from build123d import *

# Parameters (mm, degrees)
MAIN_FACE_R                    = 1.5749999999999995
MAIN_FACE_R_2                  = 1.5750000000000013
MAIN_FACE_R_3                  = 11.5
MAINFACE_DEPTH                 = 7.5
SKETCH2_W                      = 7.500000000000001
SKETCH2_H                      = 42.30000000000015
SIDEPROFILE_DEPTH              = 11
NON_INTERFERING_FILLET_DEPTH   = 67.5049810164623
BASECLEARANCE_DEPTH            = 1.5
GROUDINGBOLTHOLES_DEPTH        = 68.46897435117894
GROUDINGBOLTHOLES_DEPTH_BACK   = 68.46897435117894
SKETCH5_R                      = 1.5749999999999995
BOLTACCESSHOLES_START          = -10
SKETCH5_3_R                    = 3.55
SKETCH5_3_R_2                  = 1.5749999999999995
SKETCH5_3_R_3                  = 3.5500000000000007
BOLTACCESSHOLES_DEPTH          = 47.50000000000001
HAPPYPRINTERCURVES_R           = 2
SKETCH6_W                      = 48.78690945060761
SKETCH6_H                      = 41.74981882727384
BASEPLATE_DEPTH                = 1.2
SUPPORTTORSIONBUTBREATHE_DEPTH = 67.6961957157231


with BuildPart() as part:
    # Main Face → MainFace (new body)
    with BuildSketch(Plane.XY):
        Polygon((0, 21.150000000000077), (21.150000000000077, 21.150000000000077), (21.150000000000087, 7.98e-14), (21.150000000000507, -21.149999999999572), (8.381e-14, -21.149999999999928), (-21.149999999999924, -21.149999999999928), (-21.149999999999995, -2.69e-15), (-21.149999999999856, 21.150000000000222), align=None)
        with Locations((15.499999999999996, 15.5)):
            Circle(MAIN_FACE_R, mode=Mode.SUBTRACT)
        with Locations((15.500000000000005, -15.500000000000002)):
            Circle(MAIN_FACE_R_2, mode=Mode.SUBTRACT)
        with Locations((-15.499999999999998, -15.500000000000012)):
            Circle(MAIN_FACE_R, mode=Mode.SUBTRACT)
        with Locations((-15.50000000000001, 15.49999999999999)):
            Circle(MAIN_FACE_R, mode=Mode.SUBTRACT)
        Circle(MAIN_FACE_R_3, mode=Mode.SUBTRACT)
    extrude(amount=MAINFACE_DEPTH)

    # Sketch2 → SideProfile (add)
    with BuildSketch(Plane.ZY.offset(21.149999999999995)):
        with Locations((3.7500000000000004, 2.1849e-13)):
            Rectangle(SKETCH2_W, SKETCH2_H)
        with BuildLine():
            Line((0, -21.14999999999986), (0, 21.150000000000293))
            Line((0, 21.150000000000293), (-1.771709500841494, 21.150000000000293))
            ThreePointArc((-1.7717095008414934, 21.150000000000297), (-5.828166751938932, 20.078151362319375), (-8.825687949345335, 17.14241097816094))
            ThreePointArc((-8.82568794934533, 17.142410978160935), (-20.697100679367818, 4.412586379453849), (-36.76838475660053, -2.2726737223876654))
            ThreePointArc((-36.76838475660055, -2.2726737223876654), (-39.086170348891756, -3.6262628829235943), (-40, -6.149999999999864))
            Line((-40, -6.149999999999864), (-40, -21.149999999999864))
            Line((-40, -21.149999999999864), (0, -21.149999999999856))
        make_face()
    sideprofile = extrude(amount=SIDEPROFILE_DEPTH)

    # Sketch3 → Non-interfering fillet (cut, symmetric)
    with BuildSketch(Plane(origin=(0, 21.150000000000077, 0), x_dir=(1, 0, 0), z_dir=(0, 1, 0))):
        with BuildLine():
            Line((-21.75000000000007, 0.5999999999999999), (-21.750000000000068, 41.938133152744264))
            Line((-21.750000000000068, 41.938133152744264), (-16.932175207311897, 41.938133152744264))
            Line((-16.932175207311897, 41.938133152744264), (-16.932175207311897, 2.9783080433489855))
            Line((-16.932175207311897, 2.9783080433489855), (-21.149999999999856, 0))
            ThreePointArc((-21.149999999999856, 0), (-21.574264068711923, 0.17573593128799603), (-21.75000000000007, 0.5999999999999999))
        make_face()
    non_interfering_fillet = extrude(amount=NON_INTERFERING_FILLET_DEPTH, both=True, mode=Mode.SUBTRACT)

    # Mirror1: SideProfile, Non-interfering fillet across plane
    add(sideprofile.mirror(Plane(origin=(0, 0, 0), x_dir=(0, 0, 1), z_dir=(1, 0, 0))))
    add(non_interfering_fillet.mirror(Plane(origin=(0, 0, 0), x_dir=(0, 0, 1), z_dir=(1, 0, 0))), mode=Mode.SUBTRACT)

    # Sketch4 → BaseClearance (add)
    with BuildSketch(Plane.XZ.offset(21.149999999999928)):
        with BuildLine():
            Line((21.749999999999716, -0.5999999999999999), (21.749999999999712, -39.99999999999999))
            Line((21.749999999999712, -39.99999999999999), (32.149999999999565, -40))
            Line((32.149999999999565, -40), (32.149999999999565, 7.5))
            Line((32.149999999999565, 7.5), (-32.150000000000276, 7.5))
            Line((-32.150000000000276, 7.5), (-32.150000000000276, -40))
            Line((-32.150000000000276, -40), (-21.750000000000433, -40))
            Line((-21.750000000000433, -40), (-21.75000000000043, -0.5999999999999998))
            ThreePointArc((-21.75000000000043, -0.5999999999999998), (-21.574264068712278, -0.17573593128799736), (-21.150000000000215, 0))
            Line((-21.150000000000215, 0), (21.149999999999498, 1.73e-15))
            ThreePointArc((21.149999999999498, 1.73e-15), (21.574264068711567, -0.17573593128799248), (21.749999999999716, -0.5999999999999999))
        make_face()
    extrude(amount=BASECLEARANCE_DEPTH)

    # Sketch5 → GroudingBoltHoles (cut, two sides: drawn at the far end of the back side and taken through both)
    with BuildSketch(Plane.XZ.offset(22.64999999999993).offset(-GROUDINGBOLTHOLES_DEPTH_BACK)):
        with Locations((-26.95000000000035, -4.0000000000000036)):
            Circle(SKETCH5_R)
        with Locations((-26.950000000000344, -34)):
            Circle(SKETCH5_R)
        with Locations((26.95000000000035, -33.99999999999999)):
            Circle(SKETCH5_R)
        with Locations((26.95000000000035, -3.9999999999999964)):
            Circle(SKETCH5_R)
    extrude(amount=GROUDINGBOLTHOLES_DEPTH + GROUDINGBOLTHOLES_DEPTH_BACK, mode=Mode.SUBTRACT)

    # Sketch5<3> → BoltAccessHoles (cut)
    # profile 1 of 4: a face of its own
    with BuildSketch(Plane.XZ.offset(22.64999999999993).offset(BOLTACCESSHOLES_START)):
        with Locations((-26.950000000000344, -34)):
            Circle(SKETCH5_3_R)
        with Locations((-26.950000000000344, -34)):
            Circle(SKETCH5_3_R_2, mode=Mode.SUBTRACT)
    # profile 2 of 4: a face of its own
    with BuildSketch(Plane.XZ.offset(22.64999999999993).offset(BOLTACCESSHOLES_START)):
        with Locations((-26.95000000000035, -4.0000000000000036)):
            Circle(SKETCH5_3_R_3)
    # profile 3 of 4: a face of its own
    with BuildSketch(Plane.XZ.offset(22.64999999999993).offset(BOLTACCESSHOLES_START)):
        with Locations(Location((26.95000000000035, -3.9999999999999964, 0), (0, 0, 38.879713196))):
            Circle(SKETCH5_3_R_3)
    # profile 4 of 4: a face of its own
    with BuildSketch(Plane.XZ.offset(22.64999999999993).offset(BOLTACCESSHOLES_START)):
        with Locations(Location((26.95000000000035, -33.99999999999999, 0), (0, 0, 308.755289776))):
            Circle(SKETCH5_3_R)
    extrude(amount=-BOLTACCESSHOLES_DEPTH, mode=Mode.SUBTRACT)

    # HappyPrinterCurves
    # the kernel refuses this fillet: 2 mm, written as the material it takes off along each edge
    with BuildSketch(Plane(origin=(32.1499999999999, -27.649999999999395, -40), x_dir=(0, 0, 1), z_dir=(1.29e-15, 1, 0))) as happyprintercurves_piece_1:
        with BuildLine():
            CenterArc((HAPPYPRINTERCURVES_R, -HAPPYPRINTERCURVES_R), HAPPYPRINTERCURVES_R, 90, 90)
            Line((0, -HAPPYPRINTERCURVES_R), (0, 0))
            Line((0, 0), (HAPPYPRINTERCURVES_R, 0))
        make_face()
    extrude(amount=26.49999999999942, mode=Mode.SUBTRACT)
    with BuildSketch(Plane(origin=(21.750000000000068, -1.1499999999999382, -40), x_dir=(0, 4.3e-16, 1), z_dir=(1.72e-15, -1, 4.3e-16))) as happyprintercurves_piece_2:
        with BuildLine():
            CenterArc((HAPPYPRINTERCURVES_R, -HAPPYPRINTERCURVES_R), HAPPYPRINTERCURVES_R, 90, 90)
            Line((0, -HAPPYPRINTERCURVES_R), (0, 0))
            Line((0, 0), (HAPPYPRINTERCURVES_R, 0))
        make_face()
    extrude(amount=26.49999999999963, mode=Mode.SUBTRACT)
    with BuildSketch(Plane(origin=(-32.149999999999984, -1.1499999999999737, -40), x_dir=(0, 0, 1), z_dir=(4.74e-15, -1, 0))) as happyprintercurves_piece_3:
        with BuildLine():
            CenterArc((HAPPYPRINTERCURVES_R, -HAPPYPRINTERCURVES_R), HAPPYPRINTERCURVES_R, 90, 90)
            Line((0, -HAPPYPRINTERCURVES_R), (0, 0))
            Line((0, 0), (HAPPYPRINTERCURVES_R, 0))
        make_face()
    extrude(amount=26.500000000000487, mode=Mode.SUBTRACT)
    with BuildSketch(Plane(origin=(-32.1499999999999, -27.65000000000046, 7.5), x_dir=(1, 3.89e-15, 0), z_dir=(-3.89e-15, 1, 0))) as happyprintercurves_piece_4:
        with BuildLine():
            CenterArc((HAPPYPRINTERCURVES_R, HAPPYPRINTERCURVES_R), HAPPYPRINTERCURVES_R, 180, 90)
            Line((0, HAPPYPRINTERCURVES_R), (0, 0))
            Line((0, 0), (HAPPYPRINTERCURVES_R, 0))
        make_face()
    extrude(amount=53.800000000000644, mode=Mode.SUBTRACT)
    with BuildSketch(Plane(origin=(-21.750000000000068, -27.65000000000029, -40), x_dir=(0, 0, 1), z_dir=(-1.08e-15, 1, 0))) as happyprintercurves_piece_5:
        with BuildLine():
            CenterArc((HAPPYPRINTERCURVES_R, -HAPPYPRINTERCURVES_R), HAPPYPRINTERCURVES_R, 90, 90)
            Line((0, -HAPPYPRINTERCURVES_R), (0, 0))
            Line((0, 0), (HAPPYPRINTERCURVES_R, 0))
        make_face()
    extrude(amount=26.500000000000348, mode=Mode.SUBTRACT)
    with BuildSketch(Plane(origin=(32.150000000000084, 26.150000000000183, 7.5), x_dir=(0, 0, -1), z_dir=(-2.6e-15, -1, 0))) as happyprintercurves_piece_6:
        with BuildLine():
            CenterArc((HAPPYPRINTERCURVES_R, -HAPPYPRINTERCURVES_R), HAPPYPRINTERCURVES_R, 90, 90)
            Line((0, -HAPPYPRINTERCURVES_R), (0, 0))
            Line((0, 0), (HAPPYPRINTERCURVES_R, 0))
        make_face()
    extrude(amount=53.79999999999958, mode=Mode.SUBTRACT)

    # Sketch6 → BasePlate (add)
    with BuildSketch(Plane.XZ.offset(22.64999999999993)):
        with Locations((-0.09860427356243306, -19.12509058636308)):
            Rectangle(SKETCH6_W, SKETCH6_H)
    extrude(amount=-BASEPLATE_DEPTH)

    # Sketch7 → SupportTorsionButBreathe (cut, through all)
    with BuildSketch(Plane(origin=(3.5542e-13, -21.449999999999932, 0), x_dir=(1, 1.657e-14, 0), z_dir=(-1.657e-14, 1, 0))):
        with BuildLine():
            Line((21.75000000000003, 36.768384756600554), (21.74999999999979, 26.401553875860724))
            ThreePointArc((21.74999999999979, 26.401553875860724), (-4e-15, 4.651553875860934), (-21.74999999999979, 26.401553875860724))
            Line((-21.74999999999979, 26.401553875860724), (-21.750000000000107, 36.76838475660055))
            Line((-21.750000000000107, 36.76838475660055), (-21.750000000000114, 38))
            ThreePointArc((-21.750000000000114, 38), (-22.335786437627018, 39.41421356237322), (-23.750000000000167, 40))
            Line((-23.750000000000167, 40), (-23.750000000000167, 46.1872525671472))
            Line((-23.750000000000167, 46.1872525671472), (23.749999999999964, 46.1872525671472))
            Line((23.749999999999964, 46.1872525671472), (23.749999999999964, 40))
            ThreePointArc((23.749999999999964, 40), (22.33578643762671, 39.414213562373185), (21.75000000000002, 38))
            Line((21.75000000000002, 38), (21.75000000000003, 36.768384756600554))
        make_face()
    extrude(amount=-SUPPORTTORSIONBUTBREATHE_DEPTH, mode=Mode.SUBTRACT)


solid = part.part
Read the model definition and answer for the solid it produces. Units are mm, in the model's axes. A direction names the side the tool comes from. Give positions to 0.01 mm unless a question says otherwise; leave off trailing zeros. Loops run counter-clockwise (first coordinate to the right, second up) from the corner with the lowest first, then second, coordinate; pieces in that order, holes last. Notation, with made-up numbers: (21.25, 71.5) - (48.25, 71.5) arc R7 ccw to (48.25, 77.5) - close; hole circle Ø7 at (8, 64.25). An arc over 180 degrees is marked (long way). Answer as CSV lines item,"result". Start each with the question number.
1) Which of the six approach directions +Z, -Z, +X, -X, +Y, -Y give full straight-line access (tool end or side, diameter ignored) to faces 1 (the face through (-25.042, 4.013, -1.007)), 2 (the face through (-25.448, -17.58, -3.527)), 3 (the face through (21.75, -5, -15))?
2) Straight lines are drawn through the part: L1, parallel to Z at x = -26.95, y = -15.25 (3 decimals); L2, parallel to X at y = -10.5, z = -11; L3, parallel to X at y = 13, z = -4. For each, find the intervals that lie inside material, in ascending order. Write a range as from..to.
3) Find section B-B (y = 8.5). Write down the section's boundary in (x, z), then the cut area to 3 significant figures.
4) Find section C-C (z = 4). Write down the section's boundary in (x, y) (3 decimals), then the cut area to 3 significant figures.
5) Each of these flat-tipped pins is pushed along its axis until it touches: pin 1 Ø12.5 at (x, y) = (2.5, 9) entering from -Z; pin 2 Ø4 at (x, z) = (26.95, -4) entering from +Y; pin 3 Ø3 at (x, z) = (26.95, -34) entering from -Y; pin 4 Ø8 at (x, z) = (28, -33.5) entering from +Y. Where does it stop, or does it pass through?
6) Find section D-D (x = 15.5). Write down the section's boundary in (y, z) (3 decimals).
7) Find section A-A (x = 0). Write down the section's boundary in (y, z).
8) Determine the mould class of faces 4 (the face through (16.955, 14.897, 3.698)), 5 (the face through (-31.58, -12.55, -39.4)), 6 (the face through (-26.877, -3.597, -39.061)) for opening direction Y: released by +Y, released by -Y, zero draft, split by the parting line, or undercut.
Findings below:
1,face 1,"+Y"
1,face 2,"+Y, -Y"
1,face 3,"-Z, +Y"
2,L1,"-40..-35.575, -32.425..-5.575, -2.425..7.5"
2,L2,"-32.15..-21.75, 21.75..32.15"
2,L3,"-32.15..-30.5, -23.4..-21.75, 21.75..23.4, 30.5..32.15"
3,outline,"(-32.15, -15.7) - (-21.75, -15.7) - (-21.75, -0.6) arc R0.6 cw to (-21.15, 0) - (-7.75, 0) - (-7.75, 7.5) - (-30.15, 7.5) arc R2 ccw to (-32.15, 5.5) - close; (7.75, 0) - (21.15, 0) arc R0.6 cw to (21.75, -0.6) - (21.75, -15.7) - (32.15, -15.7) - (32.15, 5.5) arc R2 ccw to (30.15, 7.5) - (7.75, 7.5) - close; hole circle Ø7.1 at (-26.95, -4); hole circle Ø7.1 at (26.95, -4)"
3,area,"612 mm^2"
4,outline,"(-32.15, -22.65) - (32.15, -22.65) - (32.15, 21.15) - (-32.15, 21.15) - close; hole circle Ø3.15 at (-15.5, -15.5); hole circle Ø3.15 at (-15.5, 15.5); hole circle Ø23 at (0, 0); hole circle Ø3.15 at (15.5, -15.5); hole circle Ø3.15 at (15.5, 15.5)"
4,area,"2,370 mm^2"
5,pin 1,"z = 0"
5,pin 2,"y = -12.65"
5,pin 3,"through"
5,pin 4,"y = -0.24"
6,outline,"(-22.65, -11.143) - (-21.45, -11.143) - (-21.45, 0) - (-17.075, 0) - (-17.075, 7.5) - (-22.65, 7.5) - close; (-13.925, 0) - (13.925, 0) - (13.925, 7.5) - (-13.925, 7.5) - close; (17.075, 0) - (21.15, 0) - (21.15, 7.5) - (17.075, 7.5) - close"
7,outline,"(-22.65, -4.65) - (-21.45, -4.65) - (-21.45, 0) - (-11.5, 0) - (-11.5, 7.5) - (-22.65, 7.5) - close; (11.5, 0) - (21.15, 0) - (21.15, 7.5) - (11.5, 7.5) - close"
8,face 4,"undercut"
8,face 5,"zero draft"
8,face 6,"released by +Y"
